```python
from build123d import *

# Parameters (mm, degrees)
SKETCH1_W           = 177.8
SKETCH1_H           = 43.18
BOSS_EXTRUDE1_DEPTH = 2.54
SKETCH2_W           = 12.192
SKETCH2_H           = 3.81
BOSS_EXTRUDE2_DEPTH = 2.54


with BuildPart() as part:
    # Sketch1 → Boss-Extrude1 (new body)
    with BuildSketch(Plane(origin=(0, 0, 0), x_dir=(1, 0, 0), z_dir=(0, 1, 0))):
        Rectangle(SKETCH1_W, SKETCH1_H)
    extrude(amount=BOSS_EXTRUDE1_DEPTH)

    # Sketch2 → Boss-Extrude2 (add)
    with BuildSketch(Plane(origin=(0, 0, 0), x_dir=(1, 0, 0), z_dir=(0, 1, 0))):
        with Locations((-57.404, 23.495)):
            Rectangle(SKETCH2_W, SKETCH2_H)
        with Locations((-82.804, 23.495)):
            Rectangle(SKETCH2_W, SKETCH2_H)
        with Locations((-32.004, 23.495)):
            Rectangle(SKETCH2_W, SKETCH2_H)
        with Locations((-6.604, 23.495)):
            Rectangle(SKETCH2_W, SKETCH2_H)
        with Locations((18.796, 23.495)):
            Rectangle(SKETCH2_W, SKETCH2_H)
        with Locations((44.196, 23.495)):
            Rectangle(SKETCH2_W, SKETCH2_H)
        with Locations((69.596, 23.495)):
            Rectangle(SKETCH2_W, SKETCH2_H)
    boss_extrude2 = extrude(amount=BOSS_EXTRUDE2_DEPTH)

    # Mirror1: Boss-Extrude2 across plane
    add(boss_extrude2.mirror(Plane.XY))


solid = part.part
```
Can you work these out from the model? Positions are in its coordinate system, mm. Give positions to 0.01 mm unless a question says otherwise; leave off trailing zeros. Write each loop counter-clockwise with the first axis right and the second up, starting at its lowest first coordinate (ties: lowest second). Pieces come first, ordered by that corner, then holes. Notation, with made-up numbers: (74, -36.5) - (115, -36.5) arc R24 cw to (115, -15.5) - close; hole circle Ø1 at (-22, 66). An arc over 180 degrees is marked (long way). Write item = value, one per line. Start each with the question number.
1. Please list where this line runs through material, in increasing order: line 1 (Z direction, x = -75, y = 1.65).
2. For pin 1 (0.8 mm diameter, centred on y = 0.5, z = 23.5, fed in from +X); pin 2 (0.8 mm diameter, centred on x = -67, y = 1.5, fed in from -Z); pin 3 (1.3 mm diameter, centred on x = 29, y = 0.5, fed in from +Z), each with a flat end and sliding along its axis, tell me the tip position at first contact or that it passes through.
3. Imagine slicing it at A-A (x = 58). Please give me the cut outline in (y, z), and give its area (3 significant figures).
Worked answers:
q1.line_1 = -21.59 to 21.59
q2.pin_1 = 75.69
q2.pin_2 = -21.59
q2.pin_3 = 21.59
q3.outline = (0, -21.59) - (2.54, -21.59) - (2.54, 21.59) - (0, 21.59) - close
q3.area = 110 mm2
